```python
from build123d import *

# Parameters (mm, degrees)
EXTRUDE_1_DEPTH     = 10
SKETCH_2_R          = 2
EXTRUDE_2_DEPTH     = 4
SKETCH_3_R          = 2
CUT_EXTRUDE_1_DEPTH = 10


with BuildPart() as part:
    # 草图1 → 凸台-拉伸1 (new body)
    with BuildSketch(Plane.XY):
        Polygon((18, -16.25), (16, -9.25), (-24, -9.25), (-24, 9.25), (24, 9.25), (24, 8.25), (37, 8.25), (37, 0.25), (43, 0.25), (43, -0.75), (48, -0.75), (48, -6.75), (43, -6.75), (43, -17.142304845), (37, -18.75), (24, -18.75), (24, -16.25), align=None)
    extrude(amount=EXTRUDE_1_DEPTH)

    # 草图2 → 凸台-拉伸2 (add)
    with BuildSketch(Plane.XZ.offset(9.25)):
        with BuildLine():
            Line((-14.593356715, 6.674685372), (-9.5, 10))
            Line((-9.5, 10), (6.5, 10))
            Line((6.5, 10), (11.593356715, 6.674685372))
            ThreePointArc((11.593356715, 6.674685372), (12.5, 5), (11.593356715, 3.325314628))
            Line((11.593356715, 3.325314628), (6.5, 0))
            Line((6.5, 0), (-9.5, 0))
            Line((-9.5, 0), (-14.593356715, 3.325314628))
            ThreePointArc((-14.593356715, 3.325314628), (-15.5, 5), (-14.593356715, 6.674685372))
        make_face()
        with Locations((-6.75, 5)):
            Circle(SKETCH_2_R, mode=Mode.SUBTRACT)
        with Locations((3.75, 5)):
            Circle(SKETCH_2_R, mode=Mode.SUBTRACT)
    extrude(amount=EXTRUDE_2_DEPTH)

    # 草图3 → 切除-拉伸1 (cut)
    with BuildSketch(Plane(origin=(0, 9.25, 0), x_dir=(1, 0, 0), z_dir=(0, 1, 0))):
        with Locations(Location((-2, -5, 0), (0, 0, 180))):
            Circle(SKETCH_3_R)
        with Locations(Location((-11, -5, 0), (0, 0, 180))):
            Circle(SKETCH_3_R)
        with Locations(Location((7, -5, 0), (0, 0, 180))):
            Circle(SKETCH_3_R)
    extrude(amount=-CUT_EXTRUDE_1_DEPTH, mode=Mode.SUBTRACT)


solid = part.part
```
Input: part model. Units: mm. Frame: model coordinates. A direction names the side the tool comes from. Round coordinates to 2 decimals unless told otherwise and drop trailing zeros. Loops run counter-clockwise (first coordinate to the right, second up) from the corner with the lowest first, then second, coordinate; pieces in that order, holes last. Notation, with made-up numbers: (85, -18.75) -> (138, -18.75) arc R17 ccw to (138, -3.75) -> close; hole circle Ø4 at (5, 58.5). An arc over 180 degrees is marked (long way). Use one line per item in the form item = value. Start each with the question number.
Item 1: Contact query for flat-ended pins moving along their axis: pin 1 Ø5 at (x, z) = (33, 4) entering from +Y; pin 2 Ø3 at (x, z) = (-11, 5) entering from +Y; pin 3 Ø2 at (y, z) = (-18, 2.5) entering from -X. Output: stop coordinate, or through.
Item 2: Section query D-D on x = 25.5. Return the cut outline in (y, z).
Item 3: Material intervals for L1, parallel to Z at x = -2, y = 3.75; L2, parallel to Y at x = 12, z = 4.5; L3, parallel to Y at x = 13, z = 8, sorted ascending. Write a range as from..to.
Item 4: Mould query, pull axis Z, two halves, no side actions, for faces 4 (the face through (-2, 4, 7)), 5 (the face through (-24, 0, 5)), 6 (the face through (-12.01, -11.22, 1.64)). Classes: pulls with the +Z half, pulls with the -Z half, needs draft (parallel to the pull), parting line crosses it, or undercut.
Item 5: Section query B-B on y = 4.25. Return the cut outline in (x, z), then the cut area to 3 significant figures.
Item 6: Section query C-C on x = 3.75. Return the cut outline in (y, z).
Item 7: Section query A-A on y = -12. Return the cut outline in (x, z).
Item 8: Set-up query: faces 1 (the face through (43, -12, 5)), 2 (the face through (9.01, -11.22, 8.36)), 3 (the face through (-7, -9.25, 5)). Return all of +Z, -Z, +X, -X, +Y, -Y with unobstructed straight access to the full face (end or side cutting, diameter ignored); none if empty.
Ans:
q1.pin_1 = 8.25
q1.pin_2 = -0.75
q1.pin_3 = 24
q2.outline = (-18.75, 0) -> (8.25, 0) -> (8.25, 10) -> (-18.75, 10) -> close
q3.L1 = 0..3, 7..10
q3.L2 = -13.25..9.25
q3.L3 = -9.25..9.25
q4.face_4 = undercut
q4.face_5 = needs draft
q4.face_6 = pulls with the -Z half
q5.outline = (-24, 0) -> (37, 0) -> (37, 10) -> (-24, 10) -> close; hole circle Ø4 at (-11, 5); hole circle Ø4 at (-2, 5); hole circle Ø4 at (7, 5)
q5.area = 572 mm^2
q6.outline = (-13.25, 0) -> (9.25, 0) -> (9.25, 10) -> (-13.25, 10) -> (-13.25, 7) -> (-9.25, 7) -> (-9.25, 3) -> (-13.25, 3) -> close
q7.outline = (-14.59, 3.33) -> (-9.5, 0) -> (6.5, 0) -> (11.59, 3.33) arc R2 ccw to (11.59, 6.67) -> (6.5, 10) -> (-9.5, 10) -> (-14.59, 6.67) arc R2 ccw to start; (16.79, 0) -> (43, 0) -> (43, 10) -> (16.79, 10) -> close; hole circle Ø4 at (-6.75, 5); hole circle Ø4 at (3.75, 5)
q8.face_1 = +Z, -Z, +X, -Y
q8.face_2 = +Z, -Y
q8.face_3 = -Y
